Can you work these out from the model? Positions are in its coordinate system, mm. Give positions to 0.01 mm unless a question says otherwise; leave off trailing zeros. Answer in a Markdown table with one row per item.
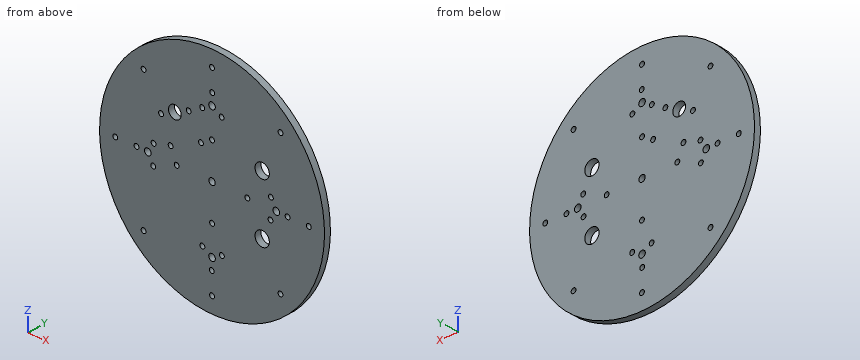
from build123d import *

# Parameters (mm, degrees)
SKETCH2_R           = 70
BOSS_EXTRUDE1_DEPTH = 4
SKETCH8_R           = 2
CUT_EXTRUDE1_DEPTH  = 100.075728612
SKETCH34_R          = 1.5
CUT_EXTRUDE8_DEPTH  = 100.075728612
CIRPATTERN7_COUNT   = 8
SKETCH56_R          = 2.05
CUT_EXTRUDE19_DEPTH = 100.075728612
SKETCH57_R          = 1.5
CUT_EXTRUDE20_DEPTH = 100.075728612
CIRPATTERN13_COUNT  = 4
SKETCH60_R          = 1.5
CUT_EXTRUDE21_DEPTH = 100.075728612
CIRPATTERN14_COUNT  = 4
SKETCH49_R          = 4.45
SKETCH49_R_2        = 3.95
CUT_EXTRUDE14_DEPTH = 100.075728612
SKETCH63_R          = 1.5
CUT_EXTRUDE24_DEPTH = 100.075728612


with BuildPart() as part:
    # Sketch2 → Boss-Extrude1 (new body)
    with BuildSketch(Plane(origin=(0, 0, 0), x_dir=(1, 0, 0), z_dir=(0, 1, 0))):
        with Locations(Location((0, 0, 0), (0, 0, 270))):
            Circle(SKETCH2_R)
    extrude(amount=BOSS_EXTRUDE1_DEPTH)

    # Sketch8 → Cut-Extrude1 (cut, through all)
    with BuildSketch(Plane(origin=(0, 4, 0), x_dir=(1, 0, 0), z_dir=(0, 1, 0))):
        with Locations(Location((0, 0, 0), (0, 0, 270))):
            Circle(SKETCH8_R)
    extrude(amount=-CUT_EXTRUDE1_DEPTH, mode=Mode.SUBTRACT)

    # Sketch34 → Cut-Extrude8 (cut, through all)
    with BuildSketch(Plane(origin=(0, 4, 0), x_dir=(1, 0, 0), z_dir=(0, 1, 0))):
        with Locations(Location((-60.25, 0, 0), (0, 0, 270))):
            Circle(SKETCH34_R)
    cut_extrude8 = extrude(amount=-CUT_EXTRUDE8_DEPTH, mode=Mode.SUBTRACT)

    # CirPattern7: Cut-Extrude8 ×8 about axis
    cirpattern7_axis = Axis((0, 0, 0), (0, 1, 0))
    for i in range(1, CIRPATTERN7_COUNT):
        add(cut_extrude8.rotate(cirpattern7_axis, i * 360 / CIRPATTERN7_COUNT), mode=Mode.SUBTRACT)

    # Sketch56 → Cut-Extrude19 (cut, through all)
    with BuildSketch(Plane(origin=(0, 4, 0), x_dir=(1, 0, 0), z_dir=(0, 1, 0))):
        with Locations(Location((0, 40, 0), (0, 0, 270))):
            Circle(SKETCH56_R)
        with Locations(Location((-40, 0, 0), (0, 0, 270))):
            Circle(SKETCH56_R)
        with Locations(Location((40, 0, 0), (0, 0, 270))):
            Circle(SKETCH56_R)
        with Locations(Location((0, -40, 0), (0, 0, 270))):
            Circle(SKETCH56_R)
    extrude(amount=-CUT_EXTRUDE19_DEPTH, mode=Mode.SUBTRACT)

    # Sketch57 → Cut-Extrude20 (cut, through all)
    with BuildSketch(Plane(origin=(0, 4, 0), x_dir=(1, 0, 0), z_dir=(0, 1, 0))):
        with Locations(Location((-36.371259829, -5.986004074, 0), (0, 0, 270))):
            Circle(SKETCH57_R)
        with Locations(Location((-46.998401681, -0.149579135, 0), (0, 0, 270))):
            Circle(SKETCH57_R)
        with Locations(Location((-36.63033849, 6.135583209, 0), (0, 0, 270))):
            Circle(SKETCH57_R)
    cut_extrude20 = extrude(amount=-CUT_EXTRUDE20_DEPTH, mode=Mode.SUBTRACT)

    # CirPattern13: Cut-Extrude20 ×4 about axis
    cirpattern13_axis = Axis((0, 0, 0), (0, 1, 0))
    for i in range(1, CIRPATTERN13_COUNT):
        add(cut_extrude20.rotate(cirpattern13_axis, i * 360 / CIRPATTERN13_COUNT), mode=Mode.SUBTRACT)

    # Sketch60 → Cut-Extrude21 (cut, through all)
    with BuildSketch(Plane(origin=(0, 4, 0), x_dir=(1, 0, 0), z_dir=(0, 1, 0))):
        with Locations(Location((22, 0, 0), (0, 0, 270))):
            Circle(SKETCH60_R)
    cut_extrude21 = extrude(amount=-CUT_EXTRUDE21_DEPTH, mode=Mode.SUBTRACT)

    # CirPattern14: Cut-Extrude21 ×4 about axis
    cirpattern14_axis = Axis((0, 0, 0), (0, 1, 0))
    for i in range(1, CIRPATTERN14_COUNT):
        add(cut_extrude21.rotate(cirpattern14_axis, i * 360 / CIRPATTERN14_COUNT), mode=Mode.SUBTRACT)

    # Sketch49 → Cut-Extrude14 (cut, through all)
    with BuildSketch(Plane.XZ):
        with Locations(Location((31.205728641, 17.95, 0), (0, 0, 270))):
            Circle(SKETCH49_R)
        with Locations(Location((31.205728641, -17.95, 0), (0, 0, 270))):
            Circle(SKETCH49_R)
        with Locations(Location((-23.140353949, 27.577599952, 0), (0, 0, 270))):
            Circle(SKETCH49_R_2)
    extrude(amount=-CUT_EXTRUDE14_DEPTH, mode=Mode.SUBTRACT)

    # Sketch63 → Cut-Extrude24 (cut, through all)
    with BuildSketch(Plane(origin=(0, 4, 0), x_dir=(1, 0, 0), z_dir=(0, 1, 0))):
        with Locations(Location((-25.789614102, -8.849040721, 0), (0, 0, 270))):
            Circle(SKETCH63_R)
        with Locations(Location((-6.889395427, -17.89855778, 0), (0, 0, 270))):
            Circle(SKETCH63_R)
        with Locations(Location((-31.731362438, -23.464183107, 0), (0, 0, 270))):
            Circle(SKETCH63_R)
        with Locations(Location((-14.54934546, -31.691016798, 0), (0, 0, 270))):
            Circle(SKETCH63_R)
    extrude(amount=-CUT_EXTRUDE24_DEPTH, mode=Mode.SUBTRACT)


solid = part.part
Q1. If I drill on line 1 (X direction, y = 3.1, z = 24.5); line 2 (Z direction, x = -21.5, y = 0.45); line 3 (Z direction, x = 31.5, y = 2.85), over which ranges is the centre line in solid material (lowest first)? Write a range as [from, to].
Checked values:
| item | result |
|---|---|
| line 1 | x = [-65.57, -32.82], [-30.65, -25.62], [-20.66, 65.57] |
| line 2 | z = [-66.62, -1.41], [1.41, 23.98], [31.17, 66.62] |
| line 3 | z = [-62.51, -22.39], [-13.51, 13.51], [22.39, 62.51] |
Q2. Imagine slicing it at A-A, the plane y = 3.35. Count the separate pieces of the cut face and the enclosed holes in it, and give its area (3 significant figures).
Checked values:
| item | result |
|---|---|
| separate pieces | 1 |
| enclosed holes | 36 |
| area | 15,000 mm² |
Q3. For pin 1 (3.5 mm diameter, centred on x = -47, z = 0.15, fed in from -Y); pin 2 (1 mm diameter, centred on x = 12.5, y = 1.5, fed in from -Z); pin 3 (1 mm diameter, centred on y = 1, z = -10.5, fed in from +X); pin 4 (1.5 mm diameter, centred on y = 2, z = -39, fed in from +X), each with a flat end and sliding along its axis, tell me the tip position at first contact or that it passes through.
Checked values:
| item | result |
|---|---|
| pin 1 | stops at y = 0 |
| pin 2 | stops at z = -68.96 |
| pin 3 | stops at x = 69.28 |
| pin 4 | stops at x = 58.63 |
